Build history of the part. All positions in model axes, mm. A direction names the side the tool comes from. Give positions to 0.01 mm unless a question says otherwise; leave off trailing zeros. Order: outer loops, then holes, each group sorted by start corner. A loop starts at its lowest first (then second) coordinate and runs counter-clockwise, first axis right, second up. Notation, with made-up numbers: (35.5, -1.75) - (87.5, -1.75) arc R18 ccw to (87.5, 24.25) - close; hole circle Ø1 at (22, -29). An arc over 180 degrees is marked (long way). Use a Markdown table: item, result.
from build123d import *

# Parameters (mm, degrees)
SKETCH_1_R      = 3
EXTRUDE_1_DEPTH = 16
SKETCH_2_R      = 4
EXTRUDE_2_DEPTH = 14
EXTRUDE_START   = 23
SKETCH_3_R      = 3
EXTRUDE_3_DEPTH = 23
SKETCH_4_R      = 2.5
EXTRUDE_4_DEPTH = 40
SKETCH_7_R      = 2
EXTRUDE_5_DEPTH = 12
EXTRUDE_START_2 = 5
SKETCH_5_R      = 2.5
EXTRUDE_6_DEPTH = 5


with BuildPart() as part:
    # 草图1 → 凸台-拉伸1 (new body)
    with BuildSketch(Plane.XY):
        Circle(SKETCH_1_R)
    extrude(amount=EXTRUDE_1_DEPTH)

    # 草图2 → 凸台-拉伸2 (add)
    with BuildSketch(Plane(origin=(0, 0, 0), x_dir=(-1, 0, 0), z_dir=(0, 0, -1))):
        Circle(SKETCH_2_R)
    extrude(amount=EXTRUDE_2_DEPTH)

    # 草图3 → 凸台-拉伸3 (add)
    with BuildSketch(Plane(origin=(0, 0, -14), x_dir=(-1, 0, 0), z_dir=(0, 0, -1)).offset(EXTRUDE_START)):
        with Locations(Location((0, 0, 0), (0, 0, 180))):
            Circle(SKETCH_3_R)
    extrude(amount=-EXTRUDE_3_DEPTH)

    # 草图4 → 凸台-拉伸4 (add)
    with BuildSketch(Plane.XY.offset(16)):
        Circle(SKETCH_4_R)
    extrude(amount=EXTRUDE_4_DEPTH)

    # 草图7 → 凸台-拉伸5 (add)
    with BuildSketch(Plane.XY.offset(56)):
        Circle(SKETCH_7_R)
    extrude(amount=EXTRUDE_5_DEPTH)

    # 草图5 → 凸台-拉伸6 (add)
    with BuildSketch(Plane(origin=(0, 0, -37), x_dir=(-1, 0, 0), z_dir=(0, 0, -1)).offset(EXTRUDE_START_2)):
        with Locations(Location((0, 0, 0), (0, 0, 180))):
            Circle(SKETCH_5_R)
    extrude(amount=-EXTRUDE_6_DEPTH)


solid = part.part
1) Slice it at D-D (z = 48). Write the cut outline in (x, y), and give its area (3 significant figures).
Computed:
| item | result |
|---|---|
| outline | circle Ø5 at (0, 0) |
| area | 19.6 mm² |
2) Pin check, flat tips, straight feed: P1, Ø4, axis at x = -1, z = 55.5, coming from the +Y side; P2, Ø1.5, axis at y = -1, z = 31.5, coming from the +X side; P3, Ø2, axis at y = -2.5, z = 24.5, coming from the +X side. Stop position of each tip, or through.
Computed:
| item | result |
|---|---|
| P1 | stops at y = 2.5 |
| P2 | stops at x = 2.49 |
| P3 | stops at x = 2 |
3) Tool access for faces 1 (the flat face through (0, 0, 68)), 2 (the flat face through (-1, 3, -14)), 3 (the flat face through (-2, 2, 16)): list every direction of +Z, -Z, +X, -X, +Y, -Y with a clear straight run to the whole face (end or side of a thin tool).
Computed:
| item | result |
|---|---|
| face 1 | +Z, +X, -X, +Y, -Y |
| face 2 | -Z |
| face 3 | +Z |
4) Slice it at A-A (x = 0). Write the cut outline in (y, z).
Computed:
| item | result |
|---|---|
| outline | (-4, -14) - (-3, -14) - (-3, -37) - (-2.5, -37) - (-2.5, -42) - (2.5, -42) - (2.5, -37) - (3, -37) - (3, -14) - (4, -14) - (4, 0) - (3, 0) - (3, 16) - (2.5, 16) - (2.5, 56) - (2, 56) - (2, 68) - (-2, 68) - (-2, 56) - (-2.5, 56) - (-2.5, 16) - (-3, 16) - (-3, 0) - (-4, 0) - close |
5) Wall check: line 1 (X direction, y = -1.5, z = 55.5); line 2 (Z direction, x = -1.25, y = 3.5); line 3 (Z direction, x = 2.5, y = 1). Give the ranges that are in metal, low to high. Write a range as from..to.
Computed:
| item | result |
|---|---|
| line 1 | x = -2..2 |
| line 2 | z = -14..0 |
| line 3 | z = -37..16 |
6) Slice it at C-C (z = -21.5). Write the cut outline in (x, y).
Computed:
| item | result |
|---|---|
| outline | circle Ø6 at (0, 0) |
